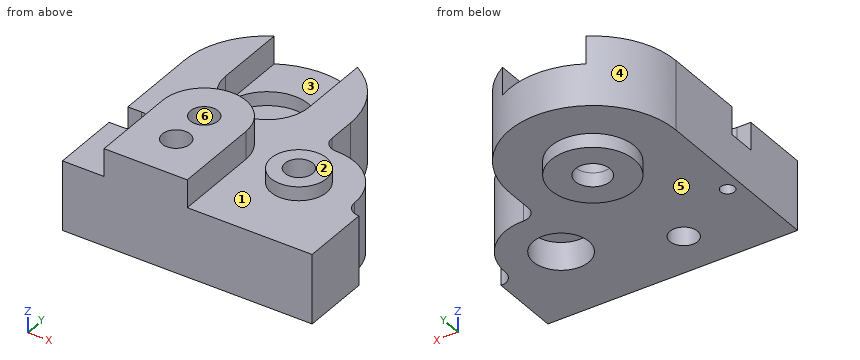
from build123d import *

# Parameters (mm, degrees)
SKETCH1_R           = 1.25
SKETCH1_R_2         = 0.5
SKETCH1_R_3         = 1
BOSS_EXTRUDE1_DEPTH = 5
SKETCH2_R           = 2
CUT_EXTRUDE1_DEPTH  = 2
CUT_EXTRUDE2_DEPTH  = 2
BOSS_EXTRUDE2_DEPTH = 2
SKETCH5_R           = 2
SKETCH5_R_2         = 1
BOSS_EXTRUDE3_DEPTH = 1
SKETCH6_R           = 1.25
BOSS_EXTRUDE4_DEPTH = 1
SKETCH7_R           = 1
CUT_EXTRUDE3_DEPTH  = 3
CUT_EXTRUDE4_DEPTH  = 2
SKETCH9_R           = 3
CUT_EXTRUDE5_DEPTH  = 1
SKETCH10_R          = 1
CUT_EXTRUDE6_DEPTH  = 4


with BuildPart() as part:
    # Sketch1 → Boss-Extrude1 (new body)
    with BuildSketch(Plane.XY):
        with BuildLine():
            Line((0, 0), (18, 0))
            Line((18, 0), (18, 5))
            ThreePointArc((18, 5), (17.292893219, 5.292893219), (17, 6))
            ThreePointArc((17, 6), (15.828427125, 8.828427125), (13, 10))
            ThreePointArc((13, 10), (12.292893219, 10.292893219), (12, 11))
            Line((12, 11), (12, 13))
            ThreePointArc((12, 13), (6, 19), (0, 13))
            Line((0, 13), (0, 0))
        make_face()
        with Locations((6, 13)):
            Circle(SKETCH1_R, mode=Mode.SUBTRACT)
        with Locations((1, 6)):
            Circle(SKETCH1_R_2, mode=Mode.SUBTRACT)
        with Locations((13, 6)):
            Circle(SKETCH1_R_3, mode=Mode.SUBTRACT)
    extrude(amount=BOSS_EXTRUDE1_DEPTH)

    # Sketch2 → Cut-Extrude1 (cut)
    with BuildSketch(Plane(origin=(0, 0, 0), x_dir=(-1, 0, 0), z_dir=(0, 0, -1))):
        with Locations((-13, 6)):
            Circle(SKETCH2_R)
    extrude(amount=-CUT_EXTRUDE1_DEPTH, mode=Mode.SUBTRACT)

    # Sketch3 → Cut-Extrude2 (cut)
    with BuildSketch(Plane.XY.offset(5)):
        with BuildLine():
            Line((3, 13), (3, 19.864652962))
            ThreePointArc((3, 19.864652962), (6, 22.864652962), (9, 19.864652962))
            Line((9, 19.864652962), (9, 13))
            ThreePointArc((9, 13), (6, 10), (3, 13))
        make_face()
    extrude(amount=-CUT_EXTRUDE2_DEPTH, mode=Mode.SUBTRACT)

    # Sketch4 → Boss-Extrude2 (add)
    with BuildSketch(Plane.XY.offset(5)):
        with BuildLine():
            Line((9, 6.266637239), (9, 0))
            Line((9, 0), (3, 0))
            Line((3, 0), (3, 6.266637239))
            ThreePointArc((3, 6.266637239), (6, 9.266637239), (9, 6.266637239))
        make_face()
    extrude(amount=BOSS_EXTRUDE2_DEPTH)

    # Sketch5 → Boss-Extrude3 (add)
    with BuildSketch(Plane.XY.offset(5)):
        with Locations((13, 6)):
            Circle(SKETCH5_R)
        with Locations((13, 6)):
            Circle(SKETCH5_R_2, mode=Mode.SUBTRACT)
    extrude(amount=BOSS_EXTRUDE3_DEPTH)

    # Sketch6 → Boss-Extrude4 (add)
    with BuildSketch(Plane(origin=(0, 0, 0), x_dir=(-1, 0, 0), z_dir=(0, 0, -1))):
        with BuildLine():
            ThreePointArc((-9, 13), (-6, 10), (-3, 13))
            ThreePointArc((-3, 13), (-6, 16), (-9, 13))
        make_face()
        with Locations((-6, 13)):
            Circle(SKETCH6_R, mode=Mode.SUBTRACT)
    extrude(amount=BOSS_EXTRUDE4_DEPTH)

    # Sketch7 → Cut-Extrude3 (cut)
    with BuildSketch(Plane.XY.offset(7)):
        with Locations((6, 6.266637239)):
            Circle(SKETCH7_R)
        with Locations((6, 3.266637239)):
            Circle(SKETCH7_R)
    extrude(amount=-CUT_EXTRUDE3_DEPTH, mode=Mode.SUBTRACT)

    # Sketch8 → Cut-Extrude4 (cut)
    with BuildSketch(Plane.XY.offset(5)):
        with BuildLine():
            Line((1, 5), (-1.045150713, 5))
            ThreePointArc((-1.045150713, 5), (-2.045150713, 6), (-1.045150713, 7))
            Line((-1.045150713, 7), (1, 7))
            ThreePointArc((1, 7), (2, 6), (1, 5))
        make_face()
    extrude(amount=-CUT_EXTRUDE4_DEPTH, mode=Mode.SUBTRACT)

    # Sketch9 → Cut-Extrude5 (cut)
    with BuildSketch(Plane.XY.offset(3)):
        with Locations((6, 13)):
            Circle(SKETCH9_R)
    extrude(amount=-CUT_EXTRUDE5_DEPTH, mode=Mode.SUBTRACT)

    # Sketch10 → Cut-Extrude6 (cut)
    with BuildSketch(Plane.XY.offset(4)):
        with Locations((6, 3.266637239)):
            Circle(SKETCH10_R)
    extrude(amount=-CUT_EXTRUDE6_DEPTH, mode=Mode.SUBTRACT)


solid = part.part
Check sheet for the modelled part. Datum: model origin and axes. Units: mm. Face numbers are marked on the shaded views. A direction names the side the tool comes from. Round coordinates to 2 decimals unless told otherwise and drop trailing zeros. Order: outer loops, then holes, each group sorted by start corner. A loop starts at its lowest first (then second) coordinate and runs counter-clockwise, first axis right, second up.
(1) Cross-section at A-A, the plane x = 6. Enter the section's corners in (y, z).
(2) Cross-section at C-C, the plane y = 1.5. Enter the section's corners in (x, z).
(3) Go/stop test with flat-tipped pins: P1, Ø1.6, axis at y = 2.5, z = 6.5, coming from the -X side; P2, Ø1.5, axis at x = 6, y = 13, coming from the -Z side; P3, Ø2, axis at y = 11.5, z = 5, coming from the -X side; P4, Ø2.5, axis at x = 13, y = 6, coming from the +Z side. Record where each tip stops, or that it passes through.
(4) Cross-section at D-D, the plane z = 1.5. Enter the section's corners in (x, y).
(5) Scan lines: probe 1 along Y at (x, z) = (6, -0.55); probe 2 along X at (y, z) = (13, 1.2); probe 3 along Y at (x, z) = (6, 1.65). Record each from-to range of solid material in increasing order.
(6) Draft check along X on the marked faces 4, 5 and 6. Enter one of: pulls with the +X half, pulls with the -X half, needs draft (parallel to the pull), parting line crosses it, or undercut.
(7) Access from +Z, -Z, +X, -X, +Y, -Y to the whole of each face (thin tool, end or side, straight path). Record for the marked faces 1, 2 and 3.
(8) Cross-section at B-B, the plane y = 6.75. Enter the section's corners in (x, z), and give its area (3 significant figures).
Check sheet entries:
1. outline: (0, 0) - (2.27, 0) - (2.27, 7) - (0, 7) - close; (4.27, 0) - (10, 0) - (10, -1) - (11.75, -1) - (11.75, 2) - (10, 2) - (10, 5) - (9.27, 5) - (9.27, 7) - (7.27, 7) - (7.27, 4) - (5.27, 4) - (5.27, 7) - (4.27, 7) - close; (14.25, -1) - (16, -1) - (16, 0) - (19, 0) - (19, 3) - (16, 3) - (16, 2) - (14.25, 2) - close
2. outline: (0, 0) - (18, 0) - (18, 5) - (9, 5) - (9, 7) - (3, 7) - (3, 5) - (0, 5) - close
3. P1: stops at x = 3
3. P2: passes through
3. P3: stops at x = 0
3. P4: stops at z = 6
4. outline: (0, 0) - (18, 0) - (18, 5) arc R1 cw to (17, 6) arc R4 ccw to (13, 10) arc R1 cw to (12, 11) - (12, 13) arc R6 ccw to (0, 13) - close; hole circle Ø1 at (1, 6); hole circle Ø2.5 at (6, 13); hole circle Ø2 at (6, 3.27); hole circle Ø4 at (13, 6)
5. probe 1: y = 10 to 11.75, 14.25 to 16
5. probe 2: x = 0 to 4.75, 7.25 to 12
5. probe 3: y = 0 to 2.27, 4.27 to 11.75, 14.25 to 19
6. face 4: parting line crosses it
6. face 5: needs draft
6. face 6: undercut
7. face 1: +Z
7. face 2: +Z, +X, +Y, -Y
7. face 3: +Z, +Y
8. outline: (0, 0) - (11.15, 0) - (11.15, 2) - (12.34, 2) - (12.34, 6) - (11.15, 6) - (11.15, 5) - (8.96, 5) - (8.96, 7) - (6.88, 7) - (6.88, 4) - (5.12, 4) - (5.12, 7) - (3.04, 7) - (3.04, 5) - (1.66, 5) - (1.66, 3) - (0, 3) - close; (13.66, 2) - (14.85, 2) - (14.85, 0) - (16.93, 0) - (16.93, 5) - (14.85, 5) - (14.85, 6) - (13.66, 6) - close
8. area: 78.9 mm2
